```python
from build123d import *

# Parameters (mm, degrees)
SKETCH1_R           = 37.5
SKETCH1_R_2         = 27.5
BOSS_EXTRUDE1_DEPTH = 50
SKETCH2_R           = 42.5
SKETCH2_R_2         = 27.5
BOSS_EXTRUDE2_DEPTH = 5
SKETCH3_R           = 2
CUT_EXTRUDE1_DEPTH  = 10


with BuildPart() as part:
    # Sketch1 → Boss-Extrude1 (new body)
    with BuildSketch(Plane.XY):
        Circle(SKETCH1_R)
        Circle(SKETCH1_R_2, mode=Mode.SUBTRACT)
    extrude(amount=BOSS_EXTRUDE1_DEPTH)

    # Sketch2 → Boss-Extrude2 (add)
    with BuildSketch(Plane.XY.offset(50)):
        Circle(SKETCH2_R)
        Circle(SKETCH2_R_2, mode=Mode.SUBTRACT)
    extrude(amount=BOSS_EXTRUDE2_DEPTH)

    # Sketch3 → Cut-Extrude1 (cut)
    with BuildSketch(Plane(origin=(0, 0, 0), x_dir=(-1, 0, 0), z_dir=(0, 0, -1))):
        with Locations((0, 32.5)):
            Circle(SKETCH3_R)
        with Locations((22.980970389, 22.980970389)):
            Circle(SKETCH3_R)
        with Locations((32.5, 0)):
            Circle(SKETCH3_R)
        with Locations((22.980970389, -22.980970389)):
            Circle(SKETCH3_R)
        with Locations((0, -32.5)):
            Circle(SKETCH3_R)
        with Locations((-22.980970389, -22.980970389)):
            Circle(SKETCH3_R)
        with Locations((-32.5, 0)):
            Circle(SKETCH3_R)
        with Locations((-22.980970389, 22.980970389)):
            Circle(SKETCH3_R)
    extrude(amount=-CUT_EXTRUDE1_DEPTH, mode=Mode.SUBTRACT)


solid = part.part
```
Verification items for the finished model (mm, model axes). A direction names the side the tool comes from. Give positions to 0.01 mm unless a question says otherwise; leave off trailing zeros. Order: outer loops, then holes, each group sorted by start corner. A loop starts at its lowest first (then second) coordinate and runs counter-clockwise, first axis right, second up. Notation, with made-up numbers: (80, 76) -> (136, 76) arc R34 cw to (136, 111) -> close; hole circle Ø9 at (88, 60). An arc over 180 degrees is marked (long way). One line per item, written item: value.
(1) Draft check along X on faces 3 (the face through (-1, -28, 55)), 4 (the face through (-32, 0, 10)), 5 (the face through (-33.727, -25.861, 52.465)). Enter one of: pulls with the +X half, pulls with the -X half, needs draft (parallel to the pull), parting line crosses it, or undercut.
Final values:
face 3: needs draft
face 4: undercut
face 5: parting line crosses it
(2) Gauge pin test, flat ends, axial feed: pin 1 (2 mm diameter, centred on x = 0, y = 32, fed in from -Z); pin 2 (6.5 mm diameter, centred on x = -22.98, y = 22.98, fed in from -Z); pin 3 (3 mm diameter, centred on x = 21, z = 15.5, fed in from -Y); pin 4 (12 mm diameter, centred on y = 5.5, z = 41, fed in from -X). Record the tip position at first contact, or that the pin passes through.
Final values:
pin 1: z = 10
pin 2: z = 0
pin 3: y = -32.03
pin 4: x = -37.5
(3) Sectioned sample at A-A on x = 0. Record the cut outline in (y, z).
Final values:
outline: (-42.5, 50) -> (-37.5, 50) -> (-37.5, 0) -> (-34.5, 0) -> (-34.5, 10) -> (-30.5, 10) -> (-30.5, 0) -> (-27.5, 0) -> (-27.5, 55) -> (-42.5, 55) -> close; (27.5, 0) -> (30.5, 0) -> (30.5, 10) -> (34.5, 10) -> (34.5, 0) -> (37.5, 0) -> (37.5, 50) -> (42.5, 50) -> (42.5, 55) -> (27.5, 55) -> close
(4) Sectioned sample at B-B on y = -19.5. Record the cut outline in (x, z).
Final values:
outline: (-37.76, 50) -> (-32.03, 50) -> (-32.03, 0) -> (-19.39, 0) -> (-19.39, 55) -> (-37.76, 55) -> close; (19.39, 0) -> (32.03, 0) -> (32.03, 50) -> (37.76, 50) -> (37.76, 55) -> (19.39, 55) -> close
(5) Tool access check on faces 1 (the face through (23, -23, 10)), 2 (the face through (-5.961, -26.846, 27.115)). Record the directions out of +Z, -Z, +X, -X, +Y, -Y that give a thin tool (end or side, any length) a straight path to the whole face; none if there is none.
Final values:
face 1: -Z
face 2: +Z, -Z
(6) Scan lines: line 1 along Y through (x, z) = (0, 4); line 2 along X through (y, z) = (1, 20.5); line 3 along Y through (x, z) = (-15.5, 15.5). Record each from-to range of solid material in increasing order. Write a range as [from, to].
Final values:
line 1: [-37.5, -34.5], [-30.5, -27.5], [27.5, 30.5], [34.5, 37.5]
line 2: [-37.49, -27.48], [27.48, 37.49]
line 3: [-34.15, -22.72], [22.72, 34.15]
(7) Sectioned sample at D-D on x = -32.5. Record the cut outline in (y, z).
Final values:
outline: (-27.39, 50) -> (-18.71, 50) -> (-18.71, 0) -> (-2, 0) -> (-2, 10) -> (2, 10) -> (2, 0) -> (18.71, 0) -> (18.71, 50) -> (27.39, 50) -> (27.39, 55) -> (-27.39, 55) -> close
(8) Sectioned sample at C-C on z = 23. Record the cut outline in (x, y), then the cut area to 3 significant figures.
Final values:
outline: circle Ø75 at (0, 0); hole circle Ø55 at (0, 0)
area: 2,040 mm^2
